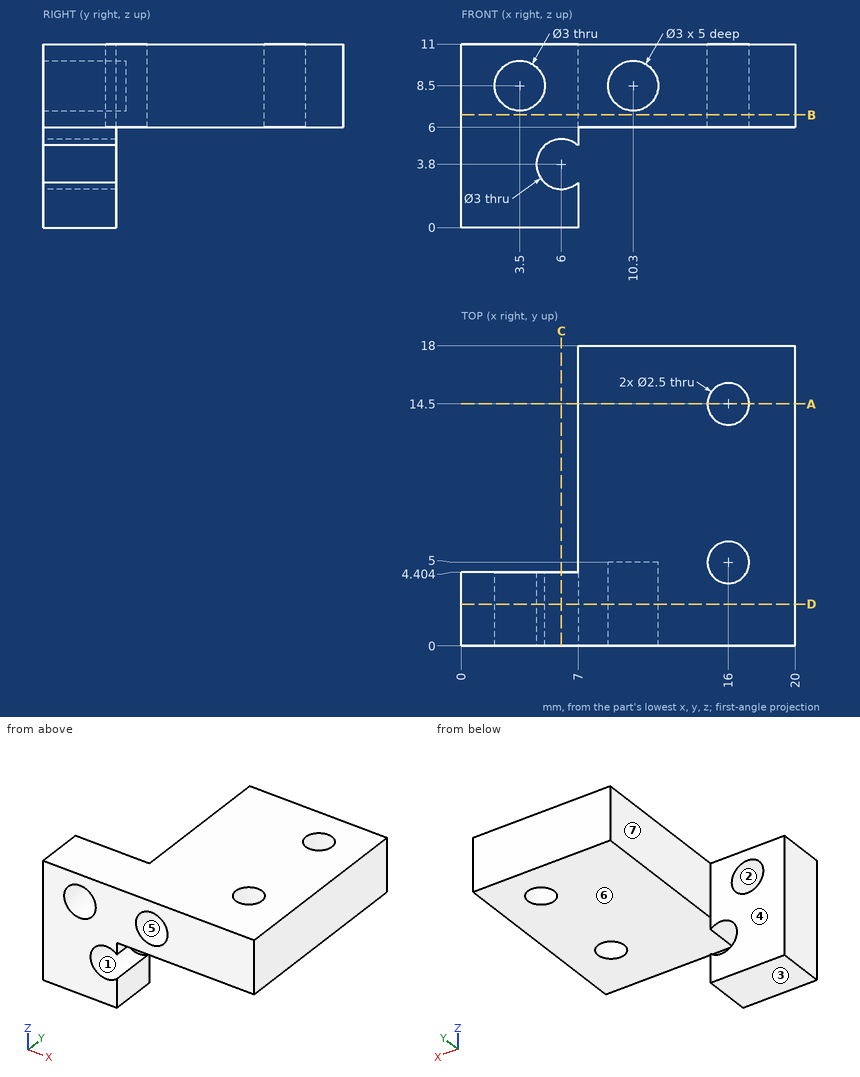
Source: three-view drawing plus pictorial views. Frame: mm from the lowest corner of the part. A direction names the side the tool comes from. Round coordinates to 2 decimals unless told otherwise and drop trailing zeros. Order: outer loops, then holes, each group sorted by start corner. A loop starts at its lowest first (then second) coordinate and runs counter-clockwise, first axis right, second up. Notation, with made-up numbers: (30, 21) -> (68, 21) arc R23 cw to (68, 43) -> close; hole circle Ø2 at (65.25, 81.5). An arc over 180 degrees is marked (long way). Use CSV: the item, a comma, the result in double quotes. Start each with the question number.
1) First-contact query: pin 1 Ø3 at (y, z) = (3, 1.5) entering from +X; pin 2 Ø1.8 at (x, z) = (3.5, 8.5) entering from -Y; pin 3 Ø3 at (x, y) = (9.5, 5.5) entering from -Z; pin 4 Ø4 at (y, z) = (8, 7.5) entering from -X. Flat tips, straight axial feed; report the tip coordinate or a pass-through.
2) Material intervals for line 1 along Y through (x, z) = (16, 9.1); line 2 along Z through (x, y) = (3.5, 1); line 3 along Z through (x, y) = (10.3, 2.35), sorted ascending. Write a range as from..to.
3) Section D-D (y = 2.5). Return the cut outline in (x, z).
4) Section C-C (x = 6). Return the cut outline in (y, z) (1 decimal).
5) Section B-B (z = 6.75). State how many separate pieces and enclosed holes the cut face has, and give its area (3 significant figures).
6) Section A-A (y = 14.5). Return the cut outline in (x, z).
7) Draft query along Z for the marked faces 1, 2, 3 and 4. Return one class per face: +Z half, -Z half, draft (parallel to the pull), parting line (faces both ways), or undercut.
8) Set-up query: the marked faces 5, 6 and 7. Return all of +Z, -Z, +X, -X, +Y, -Y with unobstructed straight access to the full face (end or side cutting, diameter ignored); none if empty.
Returned:
1,pin 1,"stops at x = 7"
1,pin 2,"passes through"
1,pin 3,"stops at z = 6"
1,pin 4,"stops at x = 7"
2,line 1,"y = 0..3.75, 6.25..13.25, 15.75..18"
2,line 2,"z = 0..7, 10..11"
2,line 3,"z = 6..7, 10..11"
3,outline,"(0, 0) -> (7, 0) -> (7, 2.68) arc R1.5 cw (long way) to (7, 4.92) -> (7, 6) -> (20, 6) -> (20, 11) -> (0, 11) -> close; hole circle Ø3 at (3.5, 8.5); hole circle Ø3 at (10.3, 8.5)"
4,outline,"(0, 0) -> (4.4, 0) -> (4.4, 2.3) -> (0, 2.3) -> close; (0, 5.3) -> (4.4, 5.3) -> (4.4, 11) -> (0, 11) -> close"
5,separate pieces,"1"
5,enclosed holes,"2"
5,area,"255 mm²"
6,outline,"(7, 6) -> (14.75, 6) -> (14.75, 11) -> (7, 11) -> close; (17.25, 6) -> (20, 6) -> (20, 11) -> (17.25, 11) -> close"
7,face 1,"undercut"
7,face 2,"undercut"
7,face 3,"-Z half"
7,face 4,"draft"
8,face 5,"-Y"
8,face 6,"-Z, +X, +Y, -Y"
8,face 7,"+Z, -Z, -X, +Y"
